Source: CAD feature listing. Evaluate the final solid. Frame: model axes, mm. A direction names the side the tool comes from. Round coordinates to 2 decimals unless told otherwise and drop trailing zeros. Write each loop counter-clockwise with the first axis right and the second up, starting at its lowest first coordinate (ties: lowest second). Pieces come first, ordered by that corner, then holes.
from build123d import *

# Parameters (mm, degrees)
EXTRUDE_1_DEPTH          = 22
SKETCH_2_R               = 8.75
CUT_EXTRUDE_1_DEPTH      = 9
CUT_EXTRUDE_3_DEPTH      = 1
CUT_EXTRUDE_3_DEPTH_BACK = 8.42975
SKETCH_4_R               = 1.9
CHAMFER_2_SIZE           = 1


with BuildPart() as part:
    # Эскиз1 → Бобышка-Вытянуть1 (new body)
    with BuildSketch(Plane.XY):
        with BuildLine():
            Line((13.201310027, -7.85542296), (13.90326512, -8.260696921))
            ThreePointArc((13.90326512, -8.260696921), (14.718656981, -4.240400213), (13.903265122, -0.220103504))
            Line((13.903265122, -0.220103504), (13.201310027, -0.625377467))
            Line((13.201310027, -0.625377467), (11.931310033, 1.574327047))
            Line((11.931310033, 1.574327047), (12.633265127, 1.979601009))
            ThreePointArc((12.633265127, 1.979601009), (9.559281984, 4.695899416), (5.669906988, 5.999897702))
            Line((5.669906988, 5.999897702), (5.669906988, 5.189349779))
            Line((5.669906988, 5.189349779), (3.129906988, 5.189349779))
            Line((3.129906988, 5.189349779), (3.129906988, 5.999897708))
            ThreePointArc((3.129906988, 5.999897708), (-0.759468012, 4.69589942), (-3.833451156, 1.979601011))
            Line((-3.833451156, 1.979601011), (-3.131496059, 1.574327046))
            Line((-3.131496059, 1.574327046), (-4.401496055, -0.625377472))
            Line((-4.401496055, -0.625377472), (-5.103451147, -0.22010351))
            ThreePointArc((-5.103451147, -0.22010351), (-5.918843009, -4.240400218), (-5.10345115, -8.260696926))
            Line((-5.10345115, -8.260696926), (-4.401496056, -7.855422963))
            Line((-4.401496056, -7.855422963), (-3.13149606, -10.055127481))
            Line((-3.13149606, -10.055127481), (-3.833451154, -10.460401444))
            ThreePointArc((-3.833451154, -10.460401444), (-0.759468012, -13.17669985), (3.129906983, -14.480698136))
            Line((3.129906983, -14.480698136), (3.129906983, -13.670150213))
            Line((3.129906983, -13.670150213), (5.669906983, -13.670150213))
            Line((5.669906983, -13.670150213), (5.669906983, -14.480698142))
            ThreePointArc((5.669906983, -14.480698142), (9.559281984, -13.176699854), (12.633265129, -10.460401443))
            Line((12.633265129, -10.460401443), (11.931310031, -10.055127478))
            Line((11.931310031, -10.055127478), (13.201310027, -7.85542296))
        make_face()
        with BuildLine():
            Line((3.15090739, -3.240400222), (5.64890659, -3.240400222))
            ThreePointArc((5.64890659, -3.240400222), (4.39990699, -5.840400222), (3.15090739, -3.240400222))
        make_face(mode=Mode.SUBTRACT)
    extrude(amount=EXTRUDE_1_DEPTH)

    # Эскиз2 → Вырез-Вытянуть1 (cut)
    with BuildSketch(Plane(origin=(0, 0, 0), x_dir=(-1, 0, 0), z_dir=(0, 0, -1))):
        with Locations((-4.39990699, -4.240400222)):
            Circle(SKETCH_2_R)
    extrude(amount=-CUT_EXTRUDE_1_DEPTH, mode=Mode.SUBTRACT)

    # Эскиз4 → Вырез-Вытянуть3 (cut, two sides: drawn at the far end of the back side and taken through both)
    with BuildSketch(Plane(origin=(0, 5.189349779, 0), x_dir=(1, 0, 0), z_dir=(0, 1, 0)).offset(-CUT_EXTRUDE_3_DEPTH_BACK)):
        with Locations(Location((4.428692677, -12.248697559, 0), (0, 0, 50.042601615))):
            Circle(SKETCH_4_R)
    extrude(amount=CUT_EXTRUDE_3_DEPTH + CUT_EXTRUDE_3_DEPTH_BACK, mode=Mode.SUBTRACT)

    # Фаска2
    chamfer_2_edges = [part.edges().sort_by_distance(p)[0] for p in [
        (4.39990699, -5.840400222, 22),
        (4.39990699, -3.240400222, 22),
        (4.39990699, -3.240400222, 9),
        (4.39990699, -5.840400222, 9),
    ]]
    chamfer(chamfer_2_edges, length=CHAMFER_2_SIZE)


solid = part.part
1) Section query C-C on x = 8.5. Return the cut outline in (y, z).
Taken from the geometry:
outline: (-13.71, 0) - (-11.97, 0) - (-11.97, 9) - (3.49, 9) - (3.49, 0) - (5.23, 0) - (5.23, 22) - (-13.71, 22) - close
2) Pull-direction query (X, two-part tool) for faces 1 (the face through (14.72, -4.3, 10.85)), 2 (the face through (4, 5.189, 5)), 3 (the face through (-0.709, 4.725, 10.846)); classes: released by +X, released by -X, zero draft, split by the parting line, or undercut.
Taken from the geometry:
face 1: released by +X
face 2: undercut
face 3: released by -X
3) Reachability of faces 4 (the face through (-3.8, -8.9, 10.8)), 5 (the face through (-3.946, -1.612, 4.437)), 6 (the face through (4.38, -2.75, 21.49)), 7 (the face through (4, -13.67, 11)) from +Z, -Z, +X, -X, +Y, -Y: full face, straight path, thin tool, end or side. Return the list, or none.
Taken from the geometry:
face 4: +Z, -Z
face 5: -Z
face 6: +Z
face 7: +Z, -Z, -Y
4) Material intervals for line 1 (Y direction, x = 12, z = 19.5); line 2 (Z direction, x = 1.75, y = -9.75); line 3 (X direction, y = -8, z = 20.5), sorted ascending.
Taken from the geometry:
line 1: y = -11.22 to -10.09, -9.94 to 1.46, 1.61 to 2.74
line 2: z = 9 to 22
line 3: x = -5.21 to -4.65, -4.32 to 13.12, 13.45 to 14.01
5) Contact query for flat-ended pins moving along their axis: P1, Ø5, axis at x = 11, z = 16, coming from the +Y side; P2, Ø1.5, axis at x = -2, z = 9.5, coming from the +Y side; P3, Ø0.9, axis at x = 4.5, z = 10.5, coming from the -Y side. Output: stop coordinate, or through.
Taken from the geometry:
P1: stops at y = 5.23
P2: stops at y = 4.39
P3: stops at y = -13.67
6) Section query D-D on y = -11. Return the cut outline in (x, z), then the cut area to 3 significant figures.
Taken from the geometry:
outline: (-3.4, 0) - (-1.16, 0) - (-1.16, 9) - (9.96, 9) - (9.96, 0) - (12.2, 0) - (12.2, 22) - (-3.4, 22) - close
area: 243 mm2
7) Section query B-B on y = 3.75. Return the cut outline in (x, z).
Taken from the geometry:
outline: (-2.13, 0) - (0.83, 0) - (0.83, 9) - (7.97, 9) - (7.97, 0) - (10.93, 0) - (10.93, 22) - (-2.13, 22) - close; hole circle Ø3.8 at (4.43, 12.25)
8) Section query A-A on z = 16.5. Return the cut outline in (x, y).
Taken from the geometry:
outline: (-5.1, -8.26) - (-4.4, -7.86) - (-3.13, -10.06) - (-3.83, -10.46) arc R10.32 ccw to (3.13, -14.48) - (3.13, -13.67) - (5.67, -13.67) - (5.67, -14.48) arc R10.32 ccw to (12.63, -10.46) - (11.93, -10.06) - (13.2, -7.86) - (13.9, -8.26) arc R10.32 ccw to (13.9, -0.22) - (13.2, -0.63) - (11.93, 1.57) - (12.63, 1.98) arc R10.32 ccw to (5.67, 6) - (5.67, 5.19) - (3.13, 5.19) - (3.13, 6) arc R10.32 ccw to (-3.83, 1.98) - (-3.13, 1.57) - (-4.4, -0.63) - (-5.1, -0.22) arc R10.32 ccw to start; hole (3.15, -3.24) arc R1.6 ccw (long way) to (5.65, -3.24) - close
